Here's how the part is built. I have some questions about the finished solid (model axes, mm). A direction names the side the tool comes from. Round coordinates to 2 decimals unless told otherwise and drop trailing zeros. Order: outer loops, then holes, each group sorted by start corner. A loop starts at its lowest first (then second) coordinate and runs counter-clockwise, first axis right, second up.
```python
from build123d import *

# Parameters (mm, degrees)
F0_R          = 15
F1_DEPTH      = 10
F3_DEPTH      = 100
F3_DEPTH_BACK = 100
F4_DEPTH      = 100
F4_DEPTH_BACK = 100
F5_R          = 4
F6_DEPTH      = 25
F7_W          = 14
F7_H          = 14
F7_R          = 4
F8_DEPTH      = 5


with BuildPart() as f1:
    # F0 (on Top) → F1 (new body)
    with BuildSketch(Plane.XY):
        Circle(F0_R)
    extrude(amount=F1_DEPTH)

    # F2 (on Front) → F3 (join, two sides)
    with BuildSketch(Plane.XZ) as f3_sk:
        with BuildLine():
            Line((19.9266501849, 9.9026951939), (-19.9266501849, 9.9026951939))
            ThreePointArc((-19.9266501849, 9.9026951939), (0, 0), (19.9266501849, 9.9026951939))
        make_face()
        with BuildLine():
            ThreePointArc((19.9266501849, 9.9026951939), (23.6977451947, 17.0365288543), (25, 25))
            ThreePointArc((25, 25), (-7.9634711457, 48.6977451947), (-19.9266501849, 9.9026951939))
            Line((-19.9266501849, 9.9026951939), (19.9266501849, 9.9026951939))
        make_face()
    extrude(amount=F3_DEPTH)
    extrude(f3_sk.sketch, amount=-F3_DEPTH_BACK)

    # F2 (on Front) → F4 (cut, two sides)
    with BuildSketch(Plane.XZ) as f4_sk:
        with BuildLine():
            ThreePointArc((-19.9266501849, 9.9026951939), (-7.9634711457, 48.6977451947), (25, 25))
            ThreePointArc((25, 25), (23.6977451947, 17.0365288543), (19.9266501849, 9.9026951939))
            Line((19.9266501849, 9.9026951939), (43.9491011202, 9.9026951939))
            Line((43.9491011202, 9.9026951939), (43.9491011202, 56.3038922846))
            Line((43.9491011202, 56.3038922846), (-35.4610793293, 56.3038922846))
            Line((-35.4610793293, 56.3038922846), (-35.4610793293, 9.9026951939))
            Line((-35.4610793293, 9.9026951939), (-19.9266501849, 9.9026951939))
        make_face()
        with BuildLine():
            ThreePointArc((19.9266501849, 9.9026951939), (23.6977451947, 17.0365288543), (25, 25))
            ThreePointArc((25, 25), (-7.9634711457, 48.6977451947), (-19.9266501849, 9.9026951939))
            Line((-19.9266501849, 9.9026951939), (19.9266501849, 9.9026951939))
        make_face()
    extrude(amount=-F4_DEPTH, mode=Mode.SUBTRACT)
    extrude(f4_sk.sketch, amount=F4_DEPTH_BACK, mode=Mode.SUBTRACT)

    # F5 (on face) → F6 (cut)
    with BuildSketch(Plane.XY.offset(9.9026951939)):
        Circle(F5_R)
    extrude(amount=-F6_DEPTH, mode=Mode.SUBTRACT)

    # F7 (on face) → F8 (cut)
    with BuildSketch(Plane(origin=(0, 0, 0), x_dir=(1, 0, 0), z_dir=(0, 0, -1))):
        Rectangle(F7_W, F7_H)
        Circle(F7_R, mode=Mode.SUBTRACT)
    extrude(amount=-F8_DEPTH, mode=Mode.SUBTRACT)


solid = f1.part
```
1) If we section it at C-C (x = 10): Write out the boundary of the cut face in (y, z), plus the area to 3 significant figures.
2) If we section it at D-D (y = 43.5): Write out the boundary of the cut face in (x, z).
3) I'm going to push flat-ended pins straight in: pin 1 (15.5 mm diameter, centred on x = 2, y = -2, fed in from -Z); pin 2 (2.5 mm diameter, centred on y = -0.5, z = 2, fed in from +X); pin 3 (1.5 mm diameter, centred on y = 13.5, z = 8.5, fed in from +X); pin 4 (4 mm diameter, centred on x = -13.5, z = 1.5, fed in from +Y). Where does each tip first touch, or does it pass through?
4) For faces 1 (the flat face through (0, -10, 0)), 2 (the flat face through (0, 7, 2)), 3 (the cylindrical face through (15, 0, 2)), 4 (the cylindrical face through (-0.867, -3.905, 7.486)), 5 (the cylindrical face through (-15, 0, 2)), which set-ups out of +Z, -Z, +X, -X, +Y, -Y let a thin tool reach every point of the face, with its end or its side?
5) If we section it at B-B (z = 1.5): Write out the boundary of the cut face in (x, y), plus the area to 3 significant figures.
6) I need wall thicknesses on line 1 (Y direction, x = 0, z = 6.05); line 2 (X direction, y = -27, z = 5); line 3 (X direction, y = 0, z = 7.3). Which ranges of each line are inside material? Lowest first, please.
7) If we section it at A-A (y = 0): Write out the boundary of the cut face in (x, z), plus the area to 3 significant figures.
Solutions:
1. outline: (-100, 2.09) - (-11.18, 2.09) - (-11.18, 0) - (11.18, 0) - (11.18, 2.09) - (100, 2.09) - (100, 9.9) - (-100, 9.9) - close
1. area: 1,610 mm2
2. outline: (-19.93, 9.9) arc R25 ccw to (19.93, 9.9) - close
3. pin 1: stops at z = 0
3. pin 2: stops at x = 15
3. pin 3: stops at x = 19.41
3. pin 4: stops at y = 9.63
4. face 1: -Z, +X, -X, +Y, -Y
4. face 2: -Z
4. face 3: -Z, +X
4. face 4: +Z, -Z
4. face 5: -Z, -X
5. outline: (-8.53, -100) - (8.53, -100) - (8.53, -12.34) arc R15 ccw to (8.53, 12.34) - (8.53, 100) - (-8.53, 100) - (-8.53, 12.34) arc R15 ccw to (-8.53, -12.34) - close; hole (-7, -7) - (7, -7) - (7, 7) - (-7, 7) - close
5. area: 3,440 mm2
6. line 1: y = -100 to -4, 4 to 100
6. line 2: x = -15 to 15
6. line 3: x = -17.66 to -4, 4 to 17.66
7. outline: (-19.93, 9.9) arc R25 ccw to (-15, 5) - (-15, 0) - (-7, 0) - (-7, 5) - (-4, 5) - (-4, 9.9) - close; (4, 5) - (7, 5) - (7, 0) - (15, 0) - (15, 5) arc R25 ccw to (19.93, 9.9) - (4, 9.9) - close
7. area: 214 mm2
